```python
from build123d import *

# Parameters (mm, degrees)
SKETCH1_W           = 27
SKETCH1_H           = 100
BOSS_EXTRUDE1_DEPTH = 60
FILLET1_R           = 10
SKETCH2_W           = 27
SKETCH2_H           = 2.5
BOSS_EXTRUDE2_DEPTH = 30
FILLET2_R           = 10
SKETCH3_R           = 8.5
CUT_EXTRUDE1_DEPTH  = 134.373535606
SKETCH4_R           = 5.5
SKETCH4_R_2         = 5
SKETCH4_R_3         = 4.5
SKETCH4_R_4         = 4
SKETCH4_R_5         = 3.5
CUT_EXTRUDE2_DEPTH  = 57


with BuildPart() as part:
    # Sketch1 → Boss-Extrude1 (new body)
    with BuildSketch(Plane.XY):
        Rectangle(SKETCH1_W, SKETCH1_H)
    extrude(amount=BOSS_EXTRUDE1_DEPTH)

    # Fillet1
    fillet1_edges = [part.edges().sort_by_distance(p)[0] for p in [
        (13.5, -50, 30),
        (-13.5, -50, 30),
    ]]
    fillet(fillet1_edges, radius=FILLET1_R)

    # Sketch2 → Boss-Extrude2 (add)
    with BuildSketch(Plane.XY.offset(60)):
        with Locations((0, 48.75)):
            Rectangle(SKETCH2_W, SKETCH2_H)
    extrude(amount=BOSS_EXTRUDE2_DEPTH)

    # Fillet2
    fillet2_edges = [part.edges().sort_by_distance(p)[0] for p in [
        (-13.5, 48.75, 90),
        (13.5, 48.75, 90),
    ]]
    fillet(fillet2_edges, radius=FILLET2_R)

    # Sketch3 → Cut-Extrude1 (cut, through all)
    with BuildSketch(Plane.XZ.offset(-47.5)):
        with Locations(Location((0, 76.5, 0), (0, 0, 270))):
            Circle(SKETCH3_R)
    extrude(amount=-CUT_EXTRUDE1_DEPTH, mode=Mode.SUBTRACT)

    # Sketch4 → Cut-Extrude2 (cut)
    with BuildSketch(Plane.XY.offset(60)):
        with Locations((0, 23.219556201)):
            Circle(SKETCH4_R)
        with Locations((0, 8.994963213)):
            Circle(SKETCH4_R_2)
        with Locations((0, -4.532345805)):
            Circle(SKETCH4_R_3)
        with Locations((0, -16.525630089)):
            Circle(SKETCH4_R_3)
        with Locations((0, -28.379457578)):
            Circle(SKETCH4_R_4)
        with Locations((0, -39.814914686)):
            Circle(SKETCH4_R_5)
    extrude(amount=-CUT_EXTRUDE2_DEPTH, mode=Mode.SUBTRACT)


solid = part.part
```
Source: CAD feature listing. Evaluate the final solid. Frame: model axes, mm. A direction names the side the tool comes from. Give positions to 0.01 mm unless a question says otherwise; leave off trailing zeros. Order: outer loops, then holes, each group sorted by start corner. A loop starts at its lowest first (then second) coordinate and runs counter-clockwise, first axis right, second up. Notation, with made-up numbers: (13.25, -8) -> (65.25, -8) arc R15 cw to (65.25, 8) -> close; hole circle Ø2 at (70, -31). An arc over 180 degrees is marked (long way). Use a Markdown table: item, result.
Q1. Section C-C (z = 22). Return the cut outline in (x, y).
A:
| item | result |
|---|---|
| outline | (-13.5, -40) arc R10 ccw to (-3.5, -50) -> (3.5, -50) arc R10 ccw to (13.5, -40) -> (13.5, 50) -> (-13.5, 50) -> close; hole circle Ø11 at (0, 23.22); hole circle Ø10 at (0, 8.99); hole circle Ø9 at (0, -16.53); hole circle Ø9 at (0, -4.53); hole circle Ø8 at (0, -28.38); hole circle Ø7 at (0, -39.81) |
Q2. Material intervals for line 1 (X direction, y = -14.5, z = 46.5); line 2 (X direction, y = 48.85, z = 76.5); line 3 (Z direction, x = -4.75, y = 19.5), sorted ascending. Write a range as [from, to].
A:
| item | result |
|---|---|
| line 1 | [-13.5, -4.02], [4.02, 13.5] |
| line 2 | [-13.5, -8.5], [8.5, 13.5] |
| line 3 | [0, 60] |
Q3. Section A-A (z = 76.5). Return the cut outline in (x, y), and give its area (3 significant figures).
A:
| item | result |
|---|---|
| outline | (-13.5, 47.5) -> (-8.5, 47.5) -> (-8.5, 50) -> (-13.5, 50) -> close; (8.5, 47.5) -> (13.5, 47.5) -> (13.5, 50) -> (8.5, 50) -> close |
| area | 25.0 mm^2 |
Q4. Section D-D (x = -6.75). Return the cut outline in (y, z).
A:
| item | result |
|---|---|
| outline | (-49.46, 0) -> (50, 0) -> (50, 71.33) -> (47.5, 71.33) -> (47.5, 60) -> (-49.46, 60) -> close; (47.5, 81.67) -> (50, 81.67) -> (50, 89.46) -> (47.5, 89.46) -> close |
Q5. Pull-direction query (Z, two-part tool) for faces 1 (the face through (3, 47.5, 68)), 2 (the face through (0, 49, 85)), 3 (the face through (0, 9, 3)); classes: +Z half, -Z half, draft (parallel to the pull), parting line (faces both ways), or undercut.
A:
| item | result |
|---|---|
| face 1 | draft |
| face 2 | undercut |
| face 3 | +Z half |
Q6. Access query for faces 4 (the face through (0, -16, 3)), 5 (the face through (0, 49, 90)). Directions: +Z, -Z, +X, -X, +Y, -Y. A direction counts if a zero-diameter tool reaches every point of the face in a straight line with its end or side. Return the directions, or none.
A:
| item | result |
|---|---|
| face 4 | +Z |
| face 5 | +Z, +X, -X, +Y, -Y |
Q7. First-contact query: P1, Ø16, axis at x = 0, y = 8.99, coming from the +Z side; P2, Ø5, axis at x = -1.5, y = 8.5, coming from the +Z side; P3, Ø5, axis at x = -8.5, z = 68, coming from the -Y side. Flat tips, straight axial feed; report the tip coordinate or a pass-through.
A:
| item | result |
|---|---|
| P1 | z = 60 |
| P2 | z = 3 |
| P3 | y = 47.5 |
